Read the model definition and answer for the solid it produces. Units are mm, in the model's axes. A direction names the side the tool comes from. Coordinates: 2 decimals unless noted, no trailing zeros. Order: outer loops, then holes, each group sorted by start corner. A loop starts at its lowest first (then second) coordinate and runs counter-clockwise, first axis right, second up. Notation, with made-up numbers: (44, 60.5) - (80, 60.5) arc R34 cw to (80, 98.5) - close; hole circle Ø1 at (55.5, 32.5). An arc over 180 degrees is marked (long way). Answer as a JSON object with one key per item and string values. Group by question number.
from build123d import *

# Parameters (mm, degrees)
F0_R     = 31.75
F1_DEPTH = 63.5
F2_R     = 29.21
F3_DEPTH = 31.75
F4_R     = 28.182549
F4_R_2   = 19.05
F5_DEPTH = 25.4


with BuildPart() as f1:
    # F0 (on Front) → F1 (new body)
    with BuildSketch(Plane.XZ):
        Circle(F0_R)
    extrude(amount=F1_DEPTH)

    # F2 (on Front) → F3 (cut)
    with BuildSketch(Plane.XZ):
        Circle(F2_R)
    extrude(amount=F3_DEPTH, mode=Mode.SUBTRACT)

    # F4 (on face) → F5 (cut)
    with BuildSketch(Plane.XZ.offset(63.5)):
        Circle(F4_R)
        Circle(F4_R_2, mode=Mode.SUBTRACT)
    extrude(amount=-F5_DEPTH, mode=Mode.SUBTRACT)


solid = f1.part
1. Straight lines are drawn through the part: L1, parallel to Z at x = 0, y = -45; L2, parallel to Z at x = 0, y = -7; L3, parallel to X at y = -40, z = -8.5. For each, find the intervals that lie inside material, in ascending order.
2. A cutting plane is placed at D-D on y = -43. Write down the section's boundary in (x, z), and give its area (3 significant figures).
3. A cutting plane is placed at A-A on x = 0. Write down the section's boundary in (y, z).
4. A cutting plane is placed at B-B on z = 0. Write down the section's boundary in (x, y), and give its area (3 significant figures).
5. Given pin 1 (6 mm diameter, centred on y = -25, z = -25, fed in from -X); pin 2 (1 mm diameter, centred on x = 11.5, y = -33.5, fed in from +Z); pin 3 (6 mm diameter, centred on x = -24.5, z = 2, fed in from -Y), each flat-ended and moving along its own axis, determine where each tip first touches the part or whether it passes through.
6. A cutting plane is placed at C-C on y = -6. Write down the section's boundary in (x, z).
7. For faces 4 (the cylindrical face through (-15.12, -50.98, -11.59)), 5 (the flat face through (-12, -63.5, -26)), 6 (the flat face through (0, -31.75, 0)), determine the directions among +Z, -Z, +X, -X, +Y, -Y from which every point of the face is accessible in a straight line to the end or side of a thin tool.
8. For a pull along X with two mould halves and no side action, classify faces 1 (the flat face through (18.4, -38.1, -5.9)), 2 (the flat face through (0, -63.5, 0)), 3 (the cylindrical face through (-6.883, -31.306, -30.995)) as pulls with the +X half, pulls with the -X half, needs draft (parallel to the pull), parting line crosses it, or undercut.
Derived:
{
 "1": {"L1": "z = -31.75 to -28.18, -19.05 to 19.05, 28.18 to 31.75", "L2": "z = -31.75 to -29.21, 29.21 to 31.75", "L3": "x = -30.59 to -26.87, -17.05 to 17.05, 26.87 to 30.59"},
 "2": {"outline": "circle Ø63.5 at (0, 0); circle Ø38.1 at (0, 0); hole circle Ø56.37 at (0, 0)", "area": "1,810 mm2"},
 "3": {"outline": "(-63.5, -31.75) - (0, -31.75) - (0, -29.21) - (-31.75, -29.21) - (-31.75, 29.21) - (0, 29.21) - (0, 31.75) - (-63.5, 31.75) - (-63.5, 28.18) - (-38.1, 28.18) - (-38.1, 19.05) - (-63.5, 19.05) - (-63.5, -19.05) - (-38.1, -19.05) - (-38.1, -28.18) - (-63.5, -28.18) - close"},
 "4": {"outline": "(-31.75, -63.5) - (-28.18, -63.5) - (-28.18, -38.1) - (-19.05, -38.1) - (-19.05, -63.5) - (19.05, -63.5) - (19.05, -38.1) - (28.18, -38.1) - (28.18, -63.5) - (31.75, -63.5) - (31.75, 0) - (29.21, 0) - (29.21, -31.75) - (-29.21, -31.75) - (-29.21, 0) - (-31.75, 0) - close", "area": "1,710 mm2"},
 "5": {"pin 1": "stops at x = -22.89", "pin 2": "stops at z = 29.78", "pin 3": "stops at y = -38.1"},
 "6": {"outline": "circle Ø63.5 at (0, 0); hole circle Ø58.42 at (0, 0)"},
 "7": {"face 4": "-Y", "face 5": "+Z, -Z, +X, -X, -Y", "face 6": "+Y"},
 "8": {"face 1": "undercut", "face 2": "needs draft", "face 3": "parting line crosses it"}
}
